from build123d import *

# Parameters (mm, degrees)
SKETCH1_W               = 40
SKETCH1_H               = 45
BOSS_EXTRUDE1_DEPTH     = 10
SKETCH2_W               = 40
SKETCH2_H               = 4
BOSS_EXTRUDE2_DEPTH     = 5
SKETCH3_W               = 4
SKETCH3_H               = 41
BOSS_EXTRUDE3_DEPTH     = 5
SKETCH4_W               = 2
SKETCH4_H               = 41
CUT_EXTRUDE1_DEPTH      = 3
SKETCH5_W               = 2
SKETCH5_H               = 20
BOSS_EXTRUDE4_DEPTH     = 15
CUT_EXTRUDE2_DEPTH      = 50.267129001
CUT_EXTRUDE2_DEPTH_BACK = 50.267129001
SKETCH8_R               = 1.5


with BuildPart() as part:
    # Sketch1 → Boss-Extrude1 (new body)
    with BuildSketch(Plane(origin=(0, 0, 0), x_dir=(1, 0, 0), z_dir=(0, 1, 0))):
        Rectangle(SKETCH1_W, SKETCH1_H)
    extrude(amount=BOSS_EXTRUDE1_DEPTH)

    # Sketch2 → Boss-Extrude2 (add)
    with BuildSketch(Plane(origin=(0, 10, 0), x_dir=(1, 0, 0), z_dir=(0, 1, 0))):
        with Locations((0, 20.5)):
            Rectangle(SKETCH2_W, SKETCH2_H)
    extrude(amount=BOSS_EXTRUDE2_DEPTH)

    # Sketch3 → Boss-Extrude3 (add)
    with BuildSketch(Plane(origin=(0, 10, 0), x_dir=(1, 0, 0), z_dir=(0, 1, 0))):
        with Locations((-18, -2)):
            Rectangle(SKETCH3_W, SKETCH3_H)
    boss_extrude3 = extrude(amount=BOSS_EXTRUDE3_DEPTH)

    # Sketch4 → Cut-Extrude1 (cut)
    with BuildSketch(Plane(origin=(0, 15, 0), x_dir=(1, 0, 0), z_dir=(0, 1, 0))):
        with Locations((-18, -2)):
            Rectangle(SKETCH4_W, SKETCH4_H)
    cut_extrude1 = extrude(amount=-CUT_EXTRUDE1_DEPTH, mode=Mode.SUBTRACT)

    # Mirror1: Boss-Extrude3, Cut-Extrude1 across plane
    add(boss_extrude3.mirror(Plane(origin=(0, 0, 0), x_dir=(0, 0, 1), z_dir=(1, 0, 0))))
    add(cut_extrude1.mirror(Plane(origin=(0, 0, 0), x_dir=(0, 0, 1), z_dir=(1, 0, 0))), mode=Mode.SUBTRACT)

    # Sketch5 → Boss-Extrude4 (add)
    with BuildSketch(Plane(origin=(0, 10, 0), x_dir=(1, 0, 0), z_dir=(0, 1, 0))):
        with Locations((-15, 8.5)):
            Rectangle(SKETCH5_W, SKETCH5_H)
    boss_extrude4 = extrude(amount=BOSS_EXTRUDE4_DEPTH)

    # Mirror2: Boss-Extrude4 across plane
    add(boss_extrude4.mirror(Plane(origin=(0, 0, 0), x_dir=(0, 0, 1), z_dir=(1, 0, 0))))

    # Sketch8 → Cut-Extrude2 (cut, two sides: drawn at the far end of the back side and taken through both)
    with BuildSketch(Plane(origin=(16, 0, 0), x_dir=(0, 0, -1), z_dir=(1, 0, 0)).offset(-CUT_EXTRUDE2_DEPTH_BACK)):
        with Locations((8.5, 20)):
            Circle(SKETCH8_R)
    extrude(amount=CUT_EXTRUDE2_DEPTH + CUT_EXTRUDE2_DEPTH_BACK, mode=Mode.SUBTRACT)


solid = part.part
Geometry check sheet. Reference: the model listing, model coordinates, mm. A direction names the side the tool comes from. Round coordinates to 2 decimals unless told otherwise and drop trailing zeros. Order: outer loops, then holes, each group sorted by start corner. A loop starts at its lowest first (then second) coordinate and runs counter-clockwise, first axis right, second up. Notation, with made-up numbers: M 58,70 L 87,70 A20 cw 87,77 Z; hole C 39,-1.5 d8. An arc over 180 degrees is marked long. Write each question's results on one line, items separated by ' | '. Start each with the question number.
1. Cross-section at C-C on x = 6. Record the boundary of the cut face in (y, z), plus the area to 3 significant figures.
2. Go/stop test with flat-tipped pins: P1, Ø1, axis at x = 4.5, z = -14, coming from the +Y side; P2, Ø10, axis at y = 19.5, z = -9, coming from the +X side; P3, Ø0.6, axis at x = 15, y = 22, coming from the -Z side; P4, Ø4, axis at x = 1, y = 13.5, coming from the +Z side. Record where each tip stops, or that it passes through.
3. Draft check along Y on faces 1 (the face through (3, 15, -20)), 2 (the face through (0, 6, 22.5)), 3 (the face through (-15.01, 21.01, -7.39)). Enter one of: pulls with the +Y half, pulls with the -Y half, needs draft (parallel to the pull), parting line crosses it, or undercut.
4. Material ranges on L1, parallel to X at y = 13.5, z = -12; L2, parallel to Z at x = 14.7, y = 20; L3, parallel to X at y = 16.75, z = 1, recorded low to high. Write a range as from..to.
5. Cross-section at D-D on z = 18. Record the boundary of the cut face in (x, y).
6. Cross-section at B-B on y = 22.25. Record the boundary of the cut face in (x, z), plus the area to 3 significant figures.
7. Set-up check for faces 4 (the face through (-16, 18, -8)), 5 (the face through (-18, 12, 2)), 6 (the face through (16, 18, -8)): record each of +Z, -Z, +X, -X, +Y, -Y from which the full face is reachable in a straight line by a thin tool's end or side.
8. Cross-section at A-A on z = -8.5. Record the boundary of the cut face in (x, y).
Resolved:
1) outline: M 0,-22.5 L 15,-22.5 L 15,-18.5 L 10,-18.5 L 10,22.5 L 0,22.5 Z | area: 470 mm2
2) P1: y = 10 | P2: x = 20 | P3: z = -18.5 | P4: z = -18.5
3) face 1: pulls with the +Y half | face 2: needs draft | face 3: undercut
4) L1: -20..-19, -17..-14, 14..17, 19..20 | L2: -18.5..-10, -7..1.5 | L3: -16..-14, 14..16
5) outline: M -20,0 L 20,0 L 20,15 L 19,15 L 19,12 L 17,12 L 17,15 L 16,15 L 16,10 L -16,10 L -16,15 L -17,15 L -17,12 L -19,12 L -19,15 L -20,15 Z
6) outline: M -16,-18.5 L -14,-18.5 L -14,1.5 L -16,1.5 Z; M 14,-18.5 L 16,-18.5 L 16,1.5 L 14,1.5 Z | area: 80.0 mm2
7) face 4: +Z, -Z, -X, +Y | face 5: +Z, +Y | face 6: +Z, -Z, +X, +Y
8) outline: M -20,0 L 20,0 L 20,15 L 19,15 L 19,12 L 17,12 L 17,15 L 16,15 L 16,18.5 L 14,18.5 L 14,10 L -14,10 L -14,18.5 L -16,18.5 L -16,15 L -17,15 L -17,12 L -19,12 L -19,15 L -20,15 Z; M -16,21.5 L -14,21.5 L -14,25 L -16,25 Z; M 14,21.5 L 16,21.5 L 16,25 L 14,25 Z
